Design review of the part built by this model. Coordinates are the model's own, in mm. Face numbers are marked on the shaded views. Give positions to 0.01 mm unless a question says otherwise; leave off trailing zeros. Loops run counter-clockwise (first coordinate to the right, second up) from the corner with the lowest first, then second, coordinate; pieces in that order, holes last. Notation, with made-up numbers: (75, 31.5) - (91, 31.5) arc R36 cw to (91, 69.5) - close; hole circle Ø8 at (9.25, -16.5). An arc over 180 degrees is marked (long way). Put each result on its own line as item: value. Start each with the question number.
```python
from build123d import *


# Not quite as in the source:
# - a fillet or chamfer that OpenCascade refuses, or shapes differently, is made with other operations: its cross-section is extruded or revolved along the edge and cut away or added


with BuildPart() as f1:
    # F0 (on Front) → F1 (revolve)
    with BuildSketch(Plane.XZ):
        with BuildLine():
            Line((0, 0), (70.2457263553, 0))
            Line((70.2457263553, 0), (70.2457263553, 12.037278153))
            ThreePointArc((70.2457263553, 12.037278153), (54.7893275552, 29.1168470867), (70.2457263553, 46.1964160204))
            Line((70.2457263553, 46.1964160204), (70.2457263553, 63.5))
            ThreePointArc((70.2457263553, 63.5), (60.7207263553, 73.025), (70.2457263553, 82.55))
            Line((70.2457263553, 82.55), (70.2457263553, 95.25))
            ThreePointArc((70.2457263553, 95.25), (67.9381906617, 104.775), (70.2457263553, 114.3))
            Line((70.2457263553, 114.3), (70.2457263553, 127))
            Line((70.2457263553, 127), (0, 127))
            Line((0, 127), (0, 0))
        make_face()
    revolve(axis=Axis((0, 0, 63.5), (0, 0, 1)))

    # F2: chamfer of 12.7 on 3 edges, made by hand

    # F2_s1 → F2_t2 (revolve, cut)
    with BuildSketch(Plane.XZ):
        with BuildLine():
            Line((70.2457263553, 54.7860135972), (64.8028692124, 65.2082915417))
            ThreePointArc((64.8028692124, 65.2082915417), (67.2107952899, 63.9964442778), (70.2457263553, 63.5))
            Line((70.2457263553, 63.5), (70.2457263553, 54.7860135972))
        make_face()
    revolve(axis=Axis((0, 0, 63.5), (0, 0, 1)), mode=Mode.SUBTRACT)

    # F2_s3 → F2_t4 (revolve, cut)
    with BuildSketch(Plane.XZ):
        with BuildLine():
            Line((70.2457263553, 92.5546468293), (69.3712508592, 97.1857341969))
            ThreePointArc((69.3712508592, 97.1857341969), (69.6830735003, 96.4332072381), (70.2457263553, 95.25))
            Line((70.2457263553, 95.25), (70.2457263553, 92.5546468293))
        make_face()
    revolve(axis=Axis((0, 0, 95.25), (0, 0, 1)), mode=Mode.SUBTRACT)

    # F2_s5 → F2_t6 (revolve, cut)
    with BuildSketch(Plane.XZ):
        with BuildLine():
            Line((70.2457263553, 2.9576382974), (63.6728956225, 14.0818369998))
            ThreePointArc((63.6728956225, 14.0818369998), (66.6706692782, 12.7854237046), (70.2457263553, 12.037278153))
            Line((70.2457263553, 12.037278153), (70.2457263553, 2.9576382974))
        make_face()
    revolve(axis=Axis((0, 0, 12.037278153), (0, 0, 1)), mode=Mode.SUBTRACT)


solid = f1.part
```
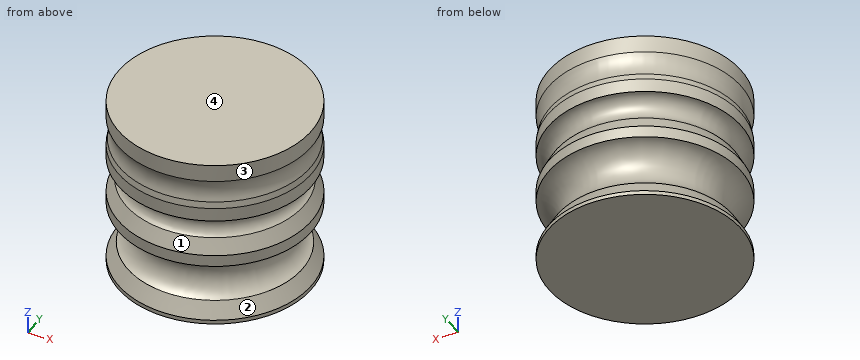
Item 1: Consider section D-D (z = 26). State the section outline as (x, y) points.
Item 2: For P1, Ø10, axis at y = 17, z = 59.5, coming from the -X side; P2, Ø5, axis at x = 10.5, z = 46.5, coming from the -Y side; P3, Ø4, axis at y = 7.5, z = 72, coming from the -X side; P4, Ø8, axis at x = -13.5, y = 3.5, coming from the -Z side, all flat-tipped, find the tip position at first contact; note any pin that passes through.
Item 3: Consider section A-A (x = 0). State the section outline as (y, z) points (3 decimals), plus the area to 3 significant figures.
Item 4: Consider section B-B (z = 90). State the section outline as (x, y) points.
Item 5: Mouldability with a two-part tool opening along Z and no side actions: class the marked faces 1, 2, 3 and 4 as pulls with the +Z half, pulls with the -Z half, needs draft (parallel to the pull), parting line crosses it, or undercut.
Item 6: For L1, parallel to Z at x = 53, y = -33.5; L2, parallel to Z at x = -51, y = -40; L3, parallel to X at y = -16, z = 98, list the stretches that pass through material, from the lowest coordinate up. Write a range as from..to.
Geometry says:
1. outline: circle Ø110.15 at (0, 0)
2. P1: stops at x = -68.56
2. P2: stops at y = -69.79
2. P3: stops at x = -60.79
2. P4: stops at z = 0
3. outline: (-70.246, 0) - (70.246, 0) - (70.246, 2.958) - (63.673, 14.082) arc R17.165 cw to (70.246, 46.196) - (70.246, 54.786) - (64.803, 65.208) arc R9.525 cw to (70.246, 82.55) - (70.246, 92.555) - (69.371, 97.186) arc R20.812 cw to (70.246, 114.3) - (70.246, 127) - (-70.246, 127) - (-70.246, 114.3) arc R20.812 cw to (-69.371, 97.186) - (-70.246, 92.555) - (-70.246, 82.55) arc R9.525 cw to (-64.803, 65.208) - (-70.246, 54.786) - (-70.246, 46.196) arc R17.165 cw to (-63.673, 14.082) - (-70.246, 2.958) - close
3. area: 16,600 mm2
4. outline: circle Ø140.49 at (0, 0)
5. face 1: undercut
5. face 2: undercut
5. face 3: needs draft
5. face 4: pulls with the +Z half
6. L1: z = 0..14.66, 43.57..67.21, 78.84..127
6. L2: z = 0..12.15, 44.73..65.18, 80.85..127
6. L3: x = -67.19..67.19
